```python
from build123d import *

# Parameters (mm, degrees)
SKETCH1_W           = 20
SKETCH1_H           = 20
SKETCH1_R           = 2.5
BOSS_EXTRUDE1_DEPTH = 2.54
SKETCH2_W           = 15.4
SKETCH2_H           = 20
SKETCH2_W_2         = 20
SKETCH2_R           = 4.6
BOSS_EXTRUDE2_DEPTH = 2.54
BOSS_EXTRUDE3_DEPTH = 20
SKETCH4_R           = 0.75
CUT_EXTRUDE1_DEPTH  = 257.103477181


with BuildPart() as part:
    # Sketch1 → Boss-Extrude1 (new body)
    with BuildSketch(Plane(origin=(0, 0, 0), x_dir=(1, 0, 0), z_dir=(0, 1, 0))):
        Rectangle(SKETCH1_W, SKETCH1_H)
        with Locations(Location((4.696699141, 4.696699141, 0), (0, 0, 270))):
            Circle(SKETCH1_R, mode=Mode.SUBTRACT)
        with Locations(Location((-4.696699141, -4.696699141, 0), (0, 0, 270))):
            Circle(SKETCH1_R, mode=Mode.SUBTRACT)
    extrude(amount=BOSS_EXTRUDE1_DEPTH)

    # Sketch2 → Boss-Extrude2 (add)
    # profile 1 of 3: a face of its own
    with BuildSketch(Plane(origin=(0, 2.54, 0), x_dir=(1, 0, 0), z_dir=(0, 1, 0))):
        with Locations((-17.7, 0)):
            Rectangle(SKETCH2_W, SKETCH2_H)
    # profile 2 of 3: a face of its own
    with BuildSketch(Plane(origin=(0, 2.54, 0), x_dir=(1, 0, 0), z_dir=(0, 1, 0))):
        Rectangle(SKETCH2_W_2, SKETCH2_H)
        with Locations(Location((-4.696699141, -4.696699141, 0), (0, 0, 270))):
            Circle(SKETCH2_R, mode=Mode.SUBTRACT)
        with Locations(Location((4.696699141, 4.696699141, 0), (0, 0, 270))):
            Circle(SKETCH2_R, mode=Mode.SUBTRACT)
    # profile 3 of 3: a face of its own
    with BuildSketch(Plane(origin=(0, 2.54, 0), x_dir=(1, 0, 0), z_dir=(0, 1, 0))):
        with Locations((17.7, 0)):
            Rectangle(SKETCH2_W, SKETCH2_H)
    extrude(amount=BOSS_EXTRUDE2_DEPTH)

    # Sketch3 → Boss-Extrude3 (add)
    with BuildSketch(Plane.XY.offset(10)):
        Polygon((-25.4, 2.54), (-25.4, 5.08), (-71.094747123, 43.964316702), (-72.740849863, 42.02990574), (-25.4, 1.744824524), (-10, 1.744824524), (-10, 2.54), align=None)
        Polygon((71.094747123, 43.964316702), (25.4, 5.08), (25.4, 2.54), (10, 2.54), (10, 1.744824524), (25.4, 1.744824524), (72.740849863, 42.02990574), align=None)
    extrude(amount=-BOSS_EXTRUDE3_DEPTH)

    # Sketch4 → Cut-Extrude1 (cut)
    with BuildSketch(Plane(origin=(-8.160655098, -9.589960753, 0), x_dir=(0.7615791187140926, -0.6480719450328537, 0), z_dir=(0.6480719450328537, 0.7615791187140926, 0))):
        with Locations(Location((-27.636315096, 4.9, 0), (0, 0, 180))):
            Circle(SKETCH4_R)
        with Locations(Location((-78.836315096, -4.9, 0), (0, 0, 180))):
            Circle(SKETCH4_R)
    cut_extrude1 = extrude(amount=-CUT_EXTRUDE1_DEPTH, mode=Mode.SUBTRACT)

    # Mirror1: Cut-Extrude1 across plane
    add(cut_extrude1.mirror(Plane(origin=(0, 0, 0), x_dir=(0, 0, 1), z_dir=(1, 0, 0))), mode=Mode.SUBTRACT)


solid = part.part
```
CAD build for the part. Positions are in the model's coordinates, mm. A direction names the side the tool comes from. Coordinates: 2 decimals unless noted, no trailing zeros. Order: outer loops, then holes, each group sorted by start corner. A loop starts at its lowest first (then second) coordinate and runs counter-clockwise, first axis right, second up. Notation, with made-up numbers: (-30.75, 63) - (-11.75, 63) arc R36 ccw to (-11.75, 100) - close; hole circle Ø9 at (28, 14.5). An arc over 180 degrees is marked (long way). Answer in a Markdown table with one row per item.
1. Flat gauge pins, fed straight in: P1, Ø4, axis at x = 46.5, z = 4, coming from the -Y side; P2, Ø0.9, axis at y = 1, z = -0.5, coming from the -X side; P3, Ø4, axis at x = -53, z = 4, coming from the -Y side; P4, Ø5.5, axis at x = -4.7, z = 4.7, coming from the -Y side. Where does each tip first touch, or does it go through?
Answer:
| item | result |
|---|---|
| P1 | y = 18 |
| P2 | x = -10 |
| P3 | y = 23.53 |
| P4 | y = 0 |
2. Pull direction Z, two halves, no side cores. Call faces 1 (the face through (0, 4, -10)), 2 (the face through (-3, 2.54, 7)), 3 (the face through (7.806, 3.792, -8.087)), 4 (the face through (0, 0, 0)): +Z half, -Z half, draft (parallel to the pull), parting line (faces both ways), or undercut.
Answer:
| item | result |
|---|---|
| face 1 | -Z half |
| face 2 | undercut |
| face 3 | undercut |
| face 4 | draft |
3. Slice it at A-A, the plane y = 37. List the corners of the cut face in (x, z), then the cut area to 3 significant figures.
Answer:
| item | result |
|---|---|
| outline | (-66.83, -10) - (-62.91, -10) - (-62.91, 10) - (-66.83, 10) - close; (62.91, -10) - (66.83, -10) - (66.83, 10) - (62.91, 10) - close |
| area | 157 mm² |
4. Slice it at B-B, the plane x = -41. List the corners of the cut face in (y, z), then the cut area to 3 significant figures.
Answer:
| item | result |
|---|---|
| outline | (15.02, -10) - (18.35, -10) - (18.35, 10) - (15.02, 10) - close |
| area | 66.7 mm² |
5. 3-axis set-ups, long thin cutter, end or side, ignore diameter. For faces 5 (the face through (48.567, 24.794, 0.14)), 6 (the face through (7, 2.54, -3)), 7 (the face through (18, 1.745, 0)): which of +Z, -Z, +X, -X, +Y, -Y reach the whole face in a straight line?
Answer:
| item | result |
|---|---|
| face 5 | +Z, -Z, +Y |
| face 6 | +Y |
| face 7 | +Z, -Z, +X, -Y |
6. Drill centre lines: L1, parallel to Y at x = -6.5, z = 1.5; L2, parallel to Y at x = 13, z = -1.5; L3, parallel to X at y = 26, z = 3. Where is each one in solid material? Low to high. Write a range as from..to.
Answer:
| item | result |
|---|---|
| L1 | 0..2.54 |
| L2 | 1.74..5.08 |
| L3 | -53.9..-49.98, 49.98..53.9 |
